Build history of the part. All positions in model axes, mm. Face numbers are marked on the shaded views. A direction names the side the tool comes from. Give positions to 0.01 mm unless a question says otherwise; leave off trailing zeros. Order: outer loops, then holes, each group sorted by start corner. A loop starts at its lowest first (then second) coordinate and runs counter-clockwise, first axis right, second up. Notation, with made-up numbers: (55, 80) -> (111, 80) arc R34 cw to (111, 115) -> close; hole circle Ø9 at (-39.75, -17). An arc over 180 degrees is marked (long way). Use a Markdown table: item, result. Add a question column.
```python
from build123d import *
from OCP.BRepFilletAPI import BRepFilletAPI_MakeChamfer
from build123d.topology import SkipClean

# Parameters (mm, degrees)
SKETCH3_W                  = 34
SKETCH3_H                  = 46
BOSS_EXTRUDE1_DEPTH        = 14
M3_CLEARANCE_HOLE1_D       = 3.4
CUT_EXTRUDE1_DEPTH         = 40.258756985
CUT_EXTRUDE1_DEPTH_BACK    = 40.258756985
SKETCH6_W                  = 12.8166
SKETCH6_H                  = 8
CUT_EXTRUDE2_DEPTH         = 38.539978689
CHAMFER1_SIZE              = 15
CHAMFER1_SIZE2             = 6.213203436
CUT_EXTRUDE3_REACH         = 39.54
BOSS_EXTRUDE2_DEPTH        = 3
FILLET1_R                  = 1
M2_5_CLEARANCE_HOLE1_D     = 2.9
M2_5_CLEARANCE_HOLE1_DEPTH = 6
FILLET2_R                  = 5


with BuildPart() as part:
    # Sketch3 → Boss-Extrude1 (new body)
    with BuildSketch(Plane(origin=(0, 0, 0), x_dir=(1, 0, 0), z_dir=(0, 1, 0))):
        with Locations((0, -9.5)):
            Rectangle(SKETCH3_W, SKETCH3_H)
    extrude(amount=-BOSS_EXTRUDE1_DEPTH)

    # M3 Clearance Hole1 (through all)
    with Locations(Plane(origin=(0, 0, 0), x_dir=(-1, 0, 0), z_dir=(0, 1, 0))):
        with Locations((7.5, 10), (7.5, -10), (-7.5, -10), (-7.5, 10)):
            Hole(M3_CLEARANCE_HOLE1_D / 2)

    # Sketch6 → Cut-Extrude1 (cut, two sides: drawn at the far end of the back side and taken through both)
    with BuildSketch(Plane(origin=(0, 0, 0), x_dir=(0, 0, -1), z_dir=(1, 0, 0)).offset(-CUT_EXTRUDE1_DEPTH_BACK)):
        with Locations((0.5917, -10)):
            Rectangle(SKETCH6_W, SKETCH6_H)
    extrude(amount=CUT_EXTRUDE1_DEPTH + CUT_EXTRUDE1_DEPTH_BACK, mode=Mode.SUBTRACT)

    # Sketch7 → Cut-Extrude2 (cut, through all)
    with BuildSketch(Plane(origin=(0, -6, 0), x_dir=(1, 0, 0), z_dir=(0, 1, 0))):
        with BuildLine():
            Line((-7.5, -26.5), (7.5, -26.5))
            Line((7.5, -26.5), (7.5, -13.8166))
            ThreePointArc((7.5, -13.8166), (3.5, -9.8166), (7.5, -5.8166))
            Line((7.5, -5.8166), (-7.5, -5.8166))
            ThreePointArc((-7.5, -5.8166), (-3.5, -9.8166), (-7.5, -13.8166))
            Line((-7.5, -13.8166), (-7.5, -26.5))
        make_face()
    extrude(amount=-CUT_EXTRUDE2_DEPTH, mode=Mode.SUBTRACT)

    # Chamfer1: one chamfer whose edges measure the first distance from different faces: ONE call of the kernel's chamfer builder (chamfer() names one face for all edges)
    chamfer1_edges_1 = [part.edges().sort_by_distance(p)[0] for p in [
        (17, -7, 32.5),
    ]]
    chamfer1_side_1 = [part.faces().sort_by_distance(p)[0] for p in [
        (17, -6.431916836, 11.410974954),
    ]]
    chamfer1_edges_2 = [part.edges().sort_by_distance(p)[0] for p in [
        (-17, -7, 32.5),
    ]]
    chamfer1_side_2 = [part.faces().sort_by_distance(p)[0] for p in [
        (-17, -6.431916836, 11.410974954),
    ]]
    chamfer1 = BRepFilletAPI_MakeChamfer(part.part.solid().wrapped)
    for e in chamfer1_edges_1:
        chamfer1.Add(CHAMFER1_SIZE, CHAMFER1_SIZE2, e.wrapped, chamfer1_side_1[0].wrapped)  # the first distance lies on this face
    for e in chamfer1_edges_2:
        chamfer1.Add(CHAMFER1_SIZE, CHAMFER1_SIZE2, e.wrapped, chamfer1_side_2[0].wrapped)  # the first distance lies on this face
    add(Compound.cast(chamfer1.Shape()), mode=Mode.REPLACE)

    # Sketch12 → Cut-Extrude3 (cut, up to next)
    with BuildSketch(Plane.XZ.offset(6), mode=Mode.PRIVATE) as cut_extrude3_sk1:
        with BuildLine():
            Line((5.940331946, 13.5), (-5.940331946, 13.5))
            ThreePointArc((-5.940331946, 13.5), (-6.704261349, 13.73665102), (-7.5, 13.8166))
            Line((-7.5, 13.8166), (-7.5, 26.5))
            Line((-7.5, 26.5), (7.5, 26.5))
            Line((7.5, 26.5), (7.5, 13.8166))
            ThreePointArc((7.5, 13.8166), (6.704261349, 13.73665102), (5.940331946, 13.5))
        make_face()
    cut_extrude3_tool1 = extrude(cut_extrude3_sk1.sketch, amount=-CUT_EXTRUDE3_REACH, mode=Mode.PRIVATE) & part.part
    add(cut_extrude3_tool1.solids().sort_by_distance((0, -6, 20.021768))[0], mode=Mode.SUBTRACT)

    # Sketch14 → Boss-Extrude2 (add)
    with SkipClean():  # the faces are left unmerged after this step: merging them gives an invalid solid
        with BuildSketch(Plane.XZ.offset(14)):
            Polygon((-17, 13.5), (-7.5, 13.5), (-7.5, 26.5), (7.5, 26.5), (7.5, 13.5), (17, 13.5), (17, 17.5), (10.786796564, 32.5), (-10.786796564, 32.5), (-17, 17.5), align=None)
        extrude(amount=BOSS_EXTRUDE2_DEPTH)

    # Fillet1
    fillet1_edges = [part.edges().sort_by_distance(p)[0] for p in [
        (-7.5, -10, 26.5),
        (7.5, -10, 26.5),
    ]]
    fillet(fillet1_edges, radius=FILLET1_R)

    # M2.5 Clearance Hole1
    with Locations(Plane.XY.offset(32.5)):
        with Locations((0, -4), (0, -14)):
            Hole(M2_5_CLEARANCE_HOLE1_D / 2, depth=M2_5_CLEARANCE_HOLE1_DEPTH)

    # Fillet2
    fillet2_edges = [part.edges().sort_by_distance(p)[0] for p in [
        (10.786796564, -7, 32.5),
        (-10.786796564, -7, 32.5),
    ]]
    fillet(fillet2_edges, radius=FILLET2_R)


solid = part.part
```
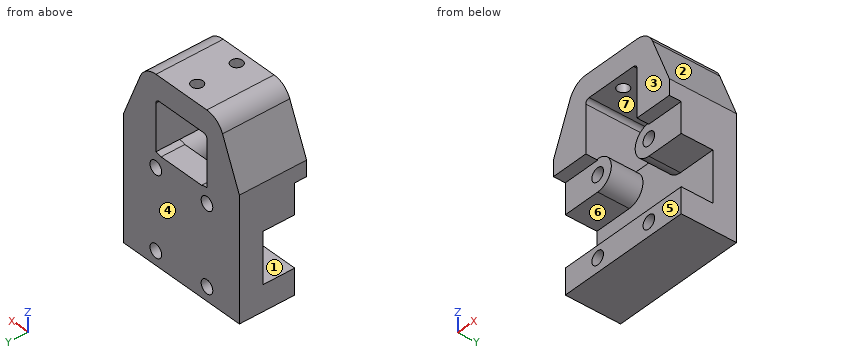
(1) Band-saw the part on B-B on x = -3. Give the cut face in (y, z), plus the area to 3 significant figures.
(2) Pin check, flat tips, straight feed: pin 1 Ø3 at (x, y) = (11.5, -3.5) entering from +Z; pin 2 Ø0.9 at (x, y) = (11.5, -15) entering from -Z; pin 3 Ø7 at (x, z) = (7.5, -9) entering from -Y. Stop position of each tip, or through.
(3) Band-saw the part on A-A on z = -10. Give the cut face in (x, y), plus the area to 3 significant figures.
(4) Band-saw the part on C-C on y = -7. Give the cut face in (x, z), plus the area to 3 significant figures.
(5) Mould opens along Z. For the marked faces 1, 2 and 3 say: released by +Z, released by -Z, zero draft, split by the parting line, or undercut.
(6) Tool access for the marked faces 4, 5, 6 and 7: list every direction of +Z, -Z, +X, -X, +Y, -Y with a clear straight run to the whole face (end or side of a thin tool).
(7) Wall check: probe 1 along Y at (x, z) = (0, 29); probe 2 along Z at (x, y) = (1, -8); probe 3 along Z at (x, y) = (-8, -7.25). Give the ranges that are in metal, low to high.
(8) Band-saw the part on D-D on z = 17. Give the cut face in (x, y).
Response:
| question | item | result |
|---|---|---|
| 1 | outline | (-17, 26.5) -> (0, 26.5) -> (0, 32.5) -> (-17, 32.5) -> close; (-14, -13.5) -> (0, -13.5) -> (0, 13.5) -> (-6, 13.5) -> (-6, -7) -> (-14, -7) -> close |
| 1 | area | 316 mm² |
| 2 | pin 1 | stops at z = 31.8 |
| 2 | pin 2 | stops at z = 13.5 |
| 2 | pin 3 | stops at y = -14 |
| 3 | outline | (-17, -14) -> (-9.2, -14) -> (-9.2, 0) -> (-17, 0) -> close; (-5.8, -14) -> (5.8, -14) -> (5.8, 0) -> (-5.8, 0) -> close; (9.2, -14) -> (17, -14) -> (17, 0) -> (9.2, 0) -> close |
| 3 | area | 381 mm² |
| 4 | outline | (-17, -13.5) -> (17, -13.5) -> (17, -7) -> (-17, -7) -> close; (-17, 5.82) -> (-7.5, 5.82) arc R4 ccw to (-7.5, 13.82) -> (-7.5, 25.5) arc R1 cw to (-6.5, 26.5) -> (6.5, 26.5) arc R1 cw to (7.5, 25.5) -> (7.5, 13.82) arc R4 ccw to (7.5, 5.82) -> (17, 5.82) -> (17, 17.5) -> (12.07, 29.41) arc R5 ccw to (7.45, 32.5) -> (-7.45, 32.5) arc R5 ccw to (-12.07, 29.41) -> (-17, 17.5) -> close; hole circle Ø3.4 at (-7.5, -10); hole circle Ø3.4 at (-7.5, 10); hole circle Ø3.4 at (7.5, -10); hole circle Ø3.4 at (7.5, 10) |
| 4 | area | 735 mm² |
| 5 | face 1 | undercut |
| 5 | face 2 | released by +Z |
| 5 | face 3 | zero draft |
| 6 | face 4 | +Z, -Z, +X, -X, +Y |
| 6 | face 5 | -Z, +X, -X, -Y |
| 6 | face 6 | +X, -X, -Y |
| 6 | face 7 | +Y, -Y |
| 7 | probe 1 | y = -17 to -15.45, -12.55 to -5.45, -2.55 to 0 |
| 7 | probe 2 | z = -13.5 to -7, 26.5 to 32.5 |
| 7 | probe 3 | z = -13.5 to -11.62, -8.38 to -7, 5.82 to 8.38, 11.62 to 32.47 |
| 8 | outline | (-17, -17) -> (-7.5, -17) -> (-7.5, 0) -> (-17, 0) -> close; (7.5, -17) -> (17, -17) -> (17, 0) -> (7.5, 0) -> close |
